Read the model definition and answer for the solid it produces. Units are mm, in the model's axes. Face numbers are marked on the shaded views. A direction names the side the tool comes from. Coordinates: 2 decimals unless noted, no trailing zeros. Write each loop counter-clockwise with the first axis right and the second up, starting at its lowest first coordinate (ties: lowest second). Pieces come first, ordered by that corner, then holes.
(1) The part is cut by section B-B, the plane x = 0. Determine the outline of the cut face in (y, z).
(2) Straight lines are drawn through the part: line 1 along Z through (x, y) = (0, -5); line 2 along X through (y, z) = (-7, -10.75). For each, find the intervals that lie inside material, in ascending order.
(3) The part is cut by section A-A, the plane z = 0. Determine the outline of the cut face in (x, y).
(4) Given pin 1 (11 mm diameter, centred on x = 0, z = 0, fed in from +Y); pin 2 (2 mm diameter, centred on y = -18, z = 7, fed in from -X); pin 3 (12 mm diameter, centred on y = -14.5, z = 0.5, fed in from -X); pin 4 (1.4 mm diameter, centred on x = -1, y = -36.5, fed in from -Z), each flat-ended and moving along its own axis, determine where each tip first touches the part or whether it passes through.
(5) The part is cut by section D-D, the plane z = 6.5. Determine the outline of the cut face in (x, y), and give its area (3 significant figures).
(6) Determine the mould class of the marked faces 4, 5, 6 and 7 for opening direction X: pulls with the +X half, pulls with the -X half, needs draft (parallel to the pull), parting line crosses it, or undercut.
(7) Which of the six approach directions +Z, -Z, +X, -X, +Y, -Y give full straight-line access (tool end or side, diameter ignored) to the marked faces 1, 2 and 3?
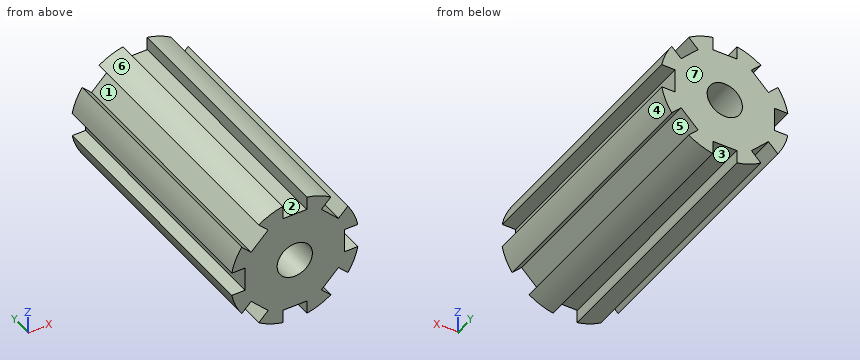
```python
from build123d import *

# Parameters (mm, degrees)
SKETCH1_R           = 12.7
BOSS_EXTRUDE1_DEPTH = 50.8
SKETCH2_R           = 3.4925
SKETCH2_W           = 4.7625
SKETCH2_H           = 5.715
SKETCH2_W_2         = 5.715
SKETCH2_H_2         = 4.7625
CUT_EXTRUDE1_DEPTH  = 109.22


with BuildPart() as part:
    # Sketch1 → Boss-Extrude1 (new body)
    with BuildSketch(Plane(origin=(0, 0, 0), x_dir=(0, 0, -1), z_dir=(0, 1, 0))):
        Circle(SKETCH1_R)
    extrude(amount=-BOSS_EXTRUDE1_DEPTH)

    # Sketch2 → Cut-Extrude1 (cut)
    with BuildSketch(Plane(origin=(0, 0, 0), x_dir=(0, 0, -1), z_dir=(0, 1, 0))):
        Circle(SKETCH2_R)
        Polygon((12.684611771, 9.317015726), (9.317015726, 12.684611771), (5.275900471, 8.643496517), (8.643496517, 5.275900471), align=None)
        with Locations((0, 12.7)):
            Rectangle(SKETCH2_W, SKETCH2_H)
        with Locations((12.7, 0)):
            Rectangle(SKETCH2_W_2, SKETCH2_H_2)
        Polygon((9.317015726, -12.684611771), (12.684611771, -9.317015726), (8.643496517, -5.275900471), (5.275900471, -8.643496517), align=None)
        with Locations((0, -12.7)):
            Rectangle(SKETCH2_W, SKETCH2_H)
        Polygon((-12.684611771, -9.317015726), (-9.317015726, -12.684611771), (-5.275900471, -8.643496517), (-8.643496517, -5.275900471), align=None)
        with Locations((-12.7, 0)):
            Rectangle(SKETCH2_W_2, SKETCH2_H_2)
        Polygon((-9.317015726, 12.684611771), (-12.684611771, 9.317015726), (-8.643496517, 5.275900471), (-5.275900471, 8.643496517), align=None)
    extrude(amount=-CUT_EXTRUDE1_DEPTH, mode=Mode.SUBTRACT)


solid = part.part
```
Computed:
1. outline: (-50.8, -9.84) - (0, -9.84) - (0, -3.49) - (-50.8, -3.49) - close; (-50.8, 3.49) - (0, 3.49) - (0, 9.84) - (-50.8, 9.84) - close
2. line 1: z = -9.84 to -3.49, 3.49 to 9.84
2. line 2: x = -6.76 to -2.38, 2.38 to 6.76
3. outline: (-9.84, -50.8) - (-3.49, -50.8) - (-3.49, 0) - (-9.84, 0) - close; (3.49, -50.8) - (9.84, -50.8) - (9.84, 0) - (3.49, 0) - close
4. pin 1: stops at y = 0
4. pin 2: stops at x = -11.19
4. pin 3: stops at x = -12.47
4. pin 4: stops at z = -9.84
5. outline: (-10.91, -50.8) - (-9.87, -50.8) - (-9.87, 0) - (-10.91, 0) - close; (-7.42, -50.8) - (7.42, -50.8) - (7.42, 0) - (-7.42, 0) - close; (9.87, -50.8) - (10.91, -50.8) - (10.91, 0) - (9.87, 0) - close
5. area: 860 mm2
6. face 4: pulls with the +X half
6. face 5: undercut
6. face 6: pulls with the -X half
6. face 7: needs draft
7. face 1: +Y, -Y
7. face 2: +Z, +Y, -Y
7. face 3: -Z, +Y, -Y
